Input: dimensioned drawing with shaded views. Units: mm. Origin: part minimum x, y, z. A direction names the side the tool comes from. Give positions to 0.01 mm unless a question says otherwise; leave off trailing zeros. Loops run counter-clockwise (first coordinate to the right, second up) from the corner with the lowest first, then second, coordinate; pieces in that order, holes last. Notation, with made-up numbers: (71.25, 12) -> (77.25, 12) arc R18 ccw to (77.25, 42) -> close; hole circle Ø1 at (-39, 78). An arc over 180 degrees is marked (long way). Answer in a Markdown table with one row per item. Add a question column.
1) Section query B-B (y = 21.5). Return the cut outline in (x, z), plus the area to 3 significant figures.
2) Draft query along X for the marked faces 4, 5 and 6. Return one class per face: +X half, -X half, draft (parallel to the pull), parting line (faces both ways), or undercut.
3) Section query A-A (z = 21). Return the cut outline in (x, y).
4) Access query for the marked faces 1, 2 and 3. Directions: +Z, -Z, +X, -X, +Y, -Y. A direction counts if a zero-diameter tool reaches every point of the face in a straight line with its end or side. Return the directions, or none.
5) First-contact query: P1, Ø12, axis at y = 22, z = 7.5, coming from the -X side; P2, Ø10, axis at x = 19, z = 19, coming from the -Y side; P3, Ø12.5, axis at y = 19.5, z = 11.5, coming from the +X side. Flat tips, straight axial feed; report the tip coordinate or a pass-through.
6) Section query D-D (z = 13). Return the cut outline in (x, y), plus the area to 3 significant figures.
7) Section query C-C (x = 19.5). Return the cut outline in (y, z), plus the area to 3 significant figures.
8) Line query: line 1 (X direction, y = 1.4, z = 21); line 2 (Z direction, x = 3, y = 1.2); line 3 (X direction, y = 22.75, z = 4). Output: solid intervals per line, ascending. Write a range as from..to.
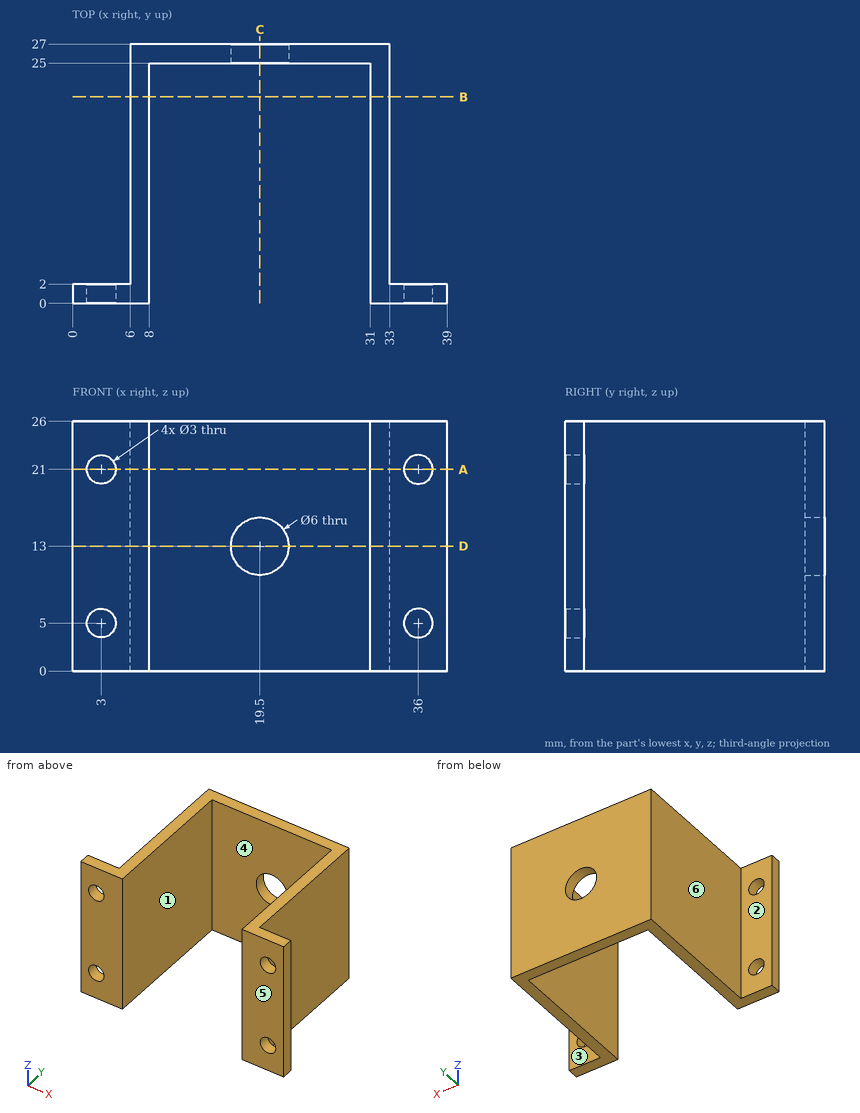
Evaluation:
| question | item | result |
|---|---|---|
| 1 | outline | (6, 0) -> (8, 0) -> (8, 26) -> (6, 26) -> close; (31, 0) -> (33, 0) -> (33, 26) -> (31, 26) -> close |
| 1 | area | 104 mm² |
| 2 | face 4 | undercut |
| 2 | face 5 | draft |
| 2 | face 6 | -X half |
| 3 | outline | (0, 0) -> (1.5, 0) -> (1.5, 2) -> (0, 2) -> close; (4.5, 0) -> (8, 0) -> (8, 25) -> (31, 25) -> (31, 0) -> (34.5, 0) -> (34.5, 2) -> (33, 2) -> (33, 27) -> (6, 27) -> (6, 2) -> (4.5, 2) -> close; (37.5, 0) -> (39, 0) -> (39, 2) -> (37.5, 2) -> close |
| 4 | face 1 | +Z, -Z, -Y |
| 4 | face 2 | +Z, -Z, -X, +Y |
| 4 | face 3 | +Z, -Z, +X, +Y |
| 5 | P1 | x = 6 |
| 5 | P2 | y = 25 |
| 5 | P3 | x = 33 |
| 6 | outline | (0, 0) -> (8, 0) -> (8, 25) -> (16.5, 25) -> (16.5, 27) -> (6, 27) -> (6, 2) -> (0, 2) -> close; (22.5, 25) -> (31, 25) -> (31, 0) -> (39, 0) -> (39, 2) -> (33, 2) -> (33, 27) -> (22.5, 27) -> close |
| 6 | area | 166 mm² |
| 7 | outline | (25, 0) -> (27, 0) -> (27, 10) -> (25, 10) -> close; (25, 16) -> (27, 16) -> (27, 26) -> (25, 26) -> close |
| 7 | area | 40.0 mm² |
| 8 | line 1 | 0..1.5, 4.5..8, 31..34.5, 37.5..39 |
| 8 | line 2 | 0..3.5, 6.5..19.5, 22.5..26 |
| 8 | line 3 | 6..8, 31..33 |
